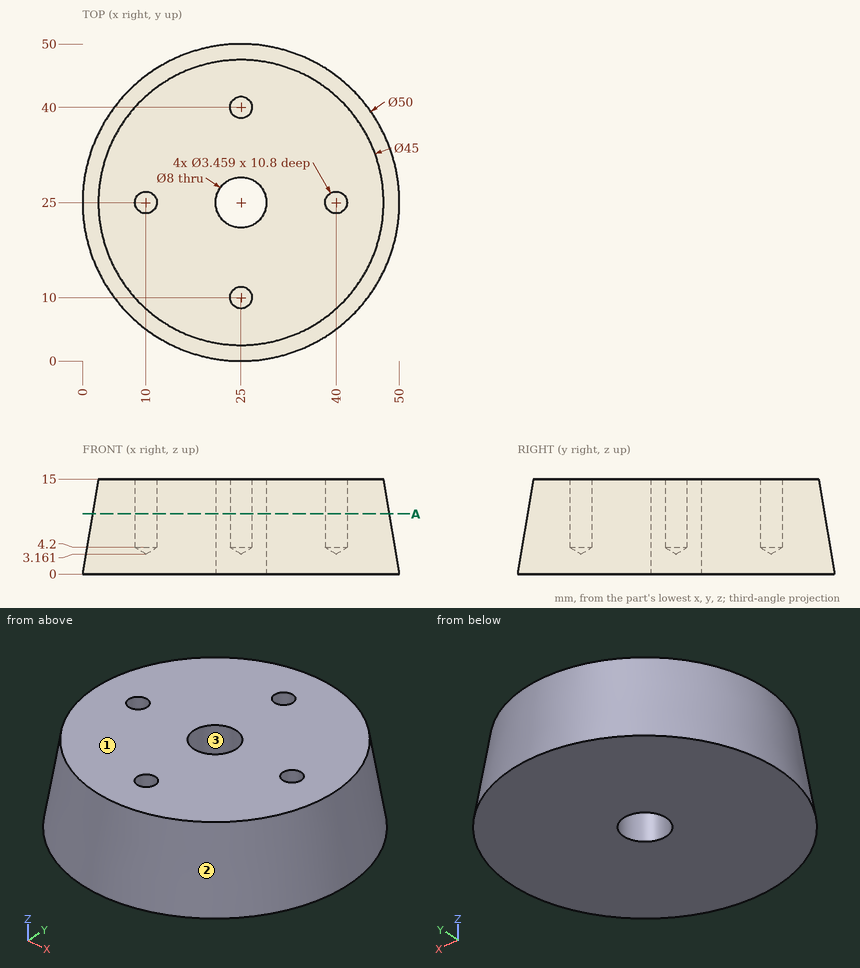
Could you check a few things on this drawing? It's one solid part, dimensions in mm from its lowest x, y, z. Coordinates: 2 decimals unless noted, no trailing zeros. Order: outer loops, then holes, each group sorted by start corner. A loop starts at its lowest first (then second) coordinate and runs counter-clockwise, first axis right, second up. Notation, with made-up numbers: (15.5, 7) - (50.5, 7) arc R19 cw to (50.5, 11) - close; hole circle Ø11 at (64, -6). An arc over 180 degrees is marked (long way). Answer as a JSON object with one key per item and string values. Group by question number.
Q1. We'd pull the mould along Y, two halves only. Please class the marked faces 1, 2 and 3: +Y half, -Y half, draft (parallel to the pull), parting line (faces both ways), or undercut.
Q2. Will these pins go through, and if not, where does the flat tip stop? P1, Ø10.5, axis at x = 25, y = 25, coming from the +Z side; P2, Ø8, axis at x = 37, z = 5.5, coming from the -Y side; P3, Ø5, axis at y = 7, z = 7, coming from the -X side; P4, Ø6, axis at x = 32.5, z = 9, coming from the -Y side.
Q3. Imagine slicing it at A-A (z = 9.5). Please give me the cut outline in (x, y).
Q4. I need wall thicknesses on line 1 (X direction, y = 24.5, z = 13.5) (1 decimal); line 2 (Y direction, x = 24.5, z = 7.75) (1 decimal); line 3 (Y direction, x = 38.5, z = 4.25) (1 decimal). Which ranges of each line are inside material? Lowest first, please. Write a range as from..to.
Determined:
{
 "1": {"face 1": "draft", "face 2": "parting line", "face 3": "undercut"},
 "2": {"P1": "stops at z = 15", "P2": "stops at y = 2.12", "P3": "stops at x = 6.83", "P4": "stops at y = 1.75"},
 "3": {"outline": "circle Ø46.83 at (25, 25); hole circle Ø3.46 at (10, 25); hole circle Ø8 at (25, 25); hole circle Ø3.46 at (25, 10); hole circle Ø3.46 at (25, 40); hole circle Ø3.46 at (40, 25)"},
 "4": {"line 1": "x = 2.3..8.3, 11.7..21, 29..38.3, 41.7..47.7", "line 2": "y = 1.3..8.3, 11.7..21, 29..38.3, 41.7..48.7", "line 3": "y = 4.8..24.1, 25.9..45.2"}
}
